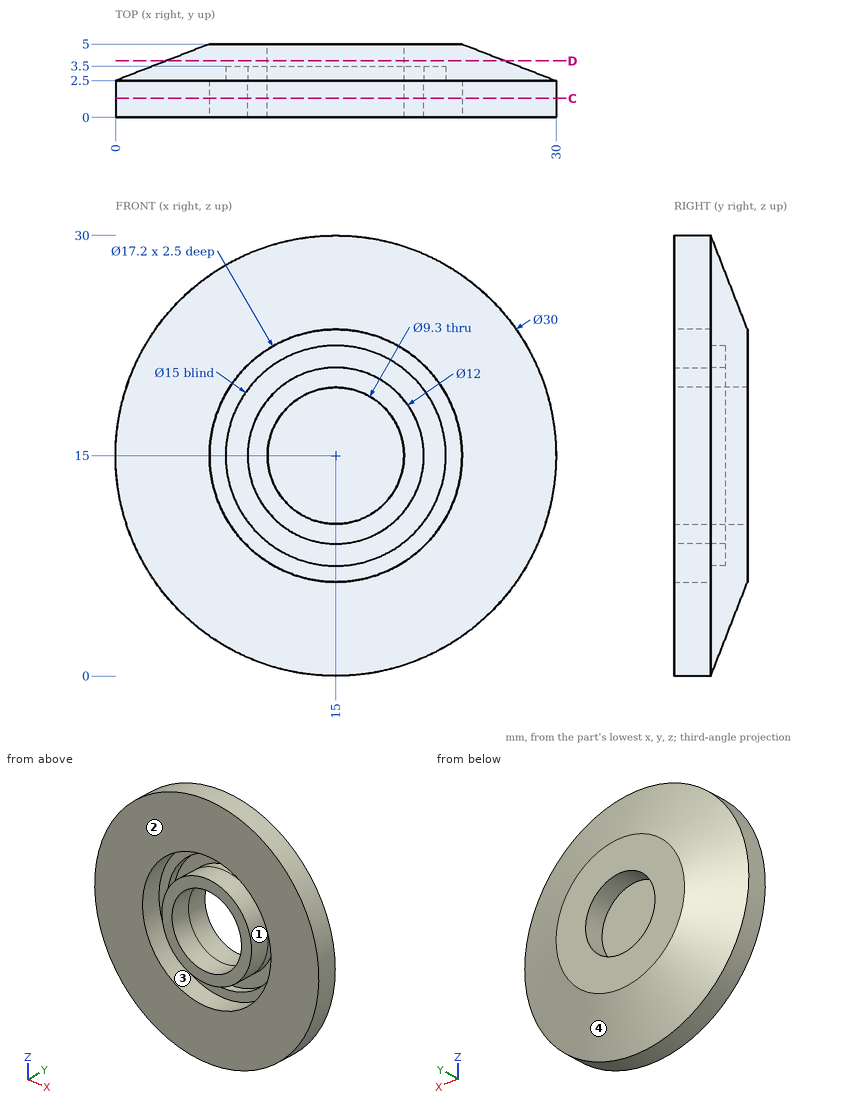
Geometry check sheet. Reference: drawing and pictorial views, mm from the part's lowest x, y, z. Round coordinates to 2 decimals unless told otherwise and drop trailing zeros. Write each loop counter-clockwise with the first axis right and the second up, starting at its lowest first coordinate (ties: lowest second). Pieces come first, ordered by that corner, then holes. Notation, with made-up numbers: (42, -28) -> (96, -28) arc R11 ccw to (96, -18) -> close; hole circle Ø4 at (52.5, -31). An arc over 180 degrees is marked (long way). Answer as CSV lines item,"result". Start each with the question number.
1) Go/stop test with flat-tipped pins: P1, Ø3, axis at x = 21.5, z = 5, coming from the +Y side; P2, Ø3, axis at x = 20, y = 3, coming from the -Z side. Record where each tip stops, or that it passes through.
2) Section check C-C on y = 1.3. Enter the section's corners in (x, z).
3) Release check for a two-part mould opening along X. For the marked faces 1, 2, 3 and 4 record: pulls with the +X half, pulls with the -X half, needs draft (parallel to the pull), parting line crosses it, or undercut.
4) Material ranges on line 1 (X direction, y = 1.75, z = 15); line 2 (Z direction, x = 18.75, y = 2.2); line 3 (Z direction, x = 14.5, y = 1.35), recorded low to high. Write a range as from..to.
5) Section check D-D on y = 3.85. Enter the section's corners in (x, z).
Found:
1,P1,"stops at y = 4.29"
1,P2,"stops at z = 0.43"
2,outline,"circle Ø30 at (15, 15); circle Ø12 at (15, 15); hole circle Ø17.2 at (15, 15); hole circle Ø9.3 at (15, 15)"
3,face 1,"undercut"
3,face 2,"needs draft"
3,face 3,"undercut"
3,face 4,"parting line crosses it"
4,line 1,"x = 0..6.4, 9..10.35, 19.65..21, 23.6..30"
4,line 2,"z = 0.48..7.26, 10.32..12.25, 17.75..19.68, 22.74..29.52"
4,line 3,"z = 0.01..6.41, 9.02..10.38, 19.62..20.98, 23.59..29.99"
5,outline,"circle Ø23.09 at (15, 15); hole circle Ø9.3 at (15, 15)"
